Autodesk Inventor part; units mm, degrees
ref_plane "YZ Plane" through (0, 0, 0) normal (1, 0, 0) x (0, 1, 0)
ref_plane "XZ Plane" through (0, 0, 0) normal (0, 1, 0) x (-1, 0, 0)
ref_plane "XY Plane" through (0, 0, 0) normal (0, 0, 1) x (1, 0, 0)
sketch "Sketch1" plane through (0, 0, 0) normal (0, 0, 1) x (1, 0, 0)
  line L0 (-34, -33) -> (34, -33)
  line L1 (34, -33) -> (34, 33)
  line L2 (34, 33) -> (-34, 33)
  line L3 (-34, 33) -> (-34, -33)
  line L4 (-34, -33) -> (34, 33) construction
  line L5 (34, -33) -> (-34, 33) construction
  point P0 (0, 0)
  dimension "d0" = 68
  dimension "d1" = 66
extrude "Extrusion1" add sketch "Sketch1" along normal blind 2
sketch "Sketch2" plane through (-34, -33, 0) normal (-1, 0, 0) x (0, 0, 1)
  line L0 (0, 0) -> (0, 66) construction
  line L1 (0, 66) -> (0, 0)
  line L2 (0, 65.9635) -> (0, 0)
  arc A0 (7.4259, 40.744) -> (0, 65.9635) centre (-222.7937, -13.3415) ccw
  arc A1 (0, 0) -> (7.4259, 40.744) centre (-36.728, 27.7427) ccw
  point P0 (0, 33)
extrude "Extrusion2" add sketch "Sketch2" against normal blind 68
sketch "Sketch3" plane through (-34, 33, 0) normal (0, 1, 0) x (1, 0, 0)
  line L0 (0, 0) -> (68, 0)
  line L1 (0, -10.0891) -> (68, -10.0891)
  line L2 (68, 0) -> (0, 0)
  line L3 (0, -2) -> (68, -2)
  line L4 (68, -2) -> (0, -2)
  line L5 (0, -2) -> (0, 0)
  line L6 (0, 0) -> (68, 0)
  line L7 (68, 0) -> (68, -2)
  arc A0 (0, 0) -> (68, 0) centre (34, 36.5643) ccw
  point P0 (34, 0)
  point P1 (51.788, -10.0891)
  point P2 (65.7135, -2)
  point P3 (2.2865, -2)
  point P4 (16.212, -10.0891)
extrude "Extrusion3" cut sketch "Sketch3" against normal blind 68 contours A0 L3 L5 | L0 A0 L3 | L7 L3 A0 | L3 A0 L1 keep common part
properties part number "Obudowa"
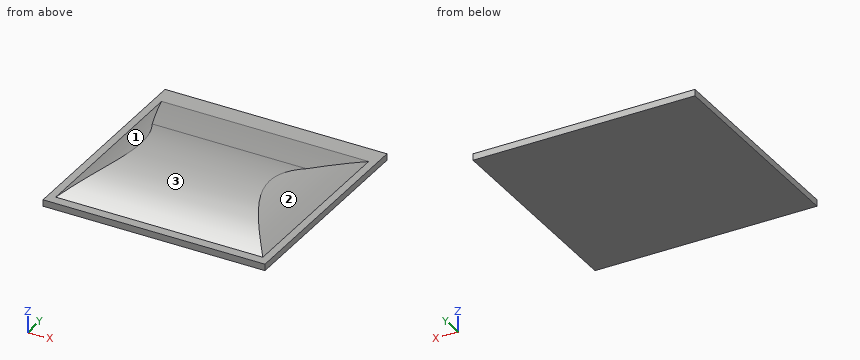
The model under review builds one solid part; all positions refer to its coordinate system, in mm. Face numbers are marked on the shaded views. Round coordinates to 2 decimals unless told otherwise and drop trailing zeros. Loops run counter-clockwise (first coordinate to the right, second up) from the corner with the lowest first, then second, coordinate; pieces in that order, holes last. Notation, with made-up numbers: (21, 23) -> (47, 23) arc R9 cw to (47, 33) -> close; hole circle Ø4 at (0, 85). An arc over 180 degrees is marked (long way). Answer in a Markdown table with one row per item.
1) Consider section C-C, the plane z = 6.25. Write out the cut boundary in (x, y), plus the area to 3 significant figures.
Taken from the geometry:
| item | result |
|---|---|
| outline | (-25.69, -21.73) -> (25.69, -21.73) -> (25.69, 12.53) -> (-25.69, 12.53) -> close |
| area | 1,760 mm² |
2) Draft analysis for pull direction X (two halves, no side actions). For the marked faces 1, 2 and 3, state which applies: pulls with the +X half, pulls with the -X half, needs draft (parallel to the pull), parting line crosses it, or undercut.
Taken from the geometry:
| item | result |
|---|---|
| face 1 | pulls with the -X half |
| face 2 | pulls with the +X half |
| face 3 | needs draft |
3) Consider section D-D, the plane x = 27. Write out the cut boundary in (y, z), plus the area to 3 significant figures.
Taken from the geometry:
| item | result |
|---|---|
| outline | (-33, 0) -> (33, 0) -> (33, 2) -> (27.1, 2) arc R236.49 ccw to (15.61, 5.44) -> (-23.72, 5.44) arc R46.03 ccw to (-30.13, 2) -> (-33, 2) -> close |
| area | 299 mm² |
4) Wall thickness on line 1 along Z through (x, y) = (4.5, -6.5); line 2 along Z through (x, y) = (-7, 2); line 3 along X through (y, z) = (-11.5, 2.5): over which ranges is each line inside the solid? List them lowest first.
Taken from the geometry:
| item | result |
|---|---|
| line 1 | z = 0 to 9.28 |
| line 2 | z = 0 to 8.72 |
| line 3 | x = -31.1 to 31.1 |
5) For pin 1 Ø6 at (x, y) = (-4.5, -9) entering from +Z; pin 2 Ø2 at (x, y) = (-25, 11) entering from +Z; pin 3 Ø4 at (x, y) = (6.5, -0.5) entering from +Z, all flat-tipped, find the tip position at first contact; note any pin that passes through.
Taken from the geometry:
| item | result |
|---|---|
| pin 1 | stops at z = 9.29 |
| pin 2 | stops at z = 6.87 |
| pin 3 | stops at z = 9.22 |
6) Consider section B-B, the plane y = 23. Write out the cut boundary in (x, z).
Taken from the geometry:
| item | result |
|---|---|
| outline | (-34, 0) -> (34, 0) -> (34, 2) -> (31.71, 2) arc R49.93 ccw to (30.06, 3.3) -> (-30.06, 3.3) arc R49.93 ccw to (-31.71, 2) -> (-34, 2) -> close |
7) Consider section A-A, the plane x = -11. Write out the cut boundary in (y, z), plus the area to 3 significant figures.
Taken from the geometry:
| item | result |
|---|---|
| outline | (-33, 0) -> (33, 0) -> (33, 2) -> (27.1, 2) arc R236.49 ccw to (7.74, 7.43) arc R46.03 ccw to (-30.13, 2) -> (-33, 2) -> close |
| area | 397 mm² |
